Geometry check sheet. Reference: drawing and pictorial views, mm from the part's lowest x, y, z. Round coordinates to 2 decimals unless told otherwise and drop trailing zeros. Order: outer loops, then holes, each group sorted by start corner. A loop starts at its lowest first (then second) coordinate and runs counter-clockwise, first axis right, second up. Notation, with made-up numbers: M -27,68 L 13,68 A18 cw 13,92 Z; hole C -16.75,23.25 d10. An arc over 180 degrees is marked long. Answer as a JSON object with one key per item and string values. Group by question number.
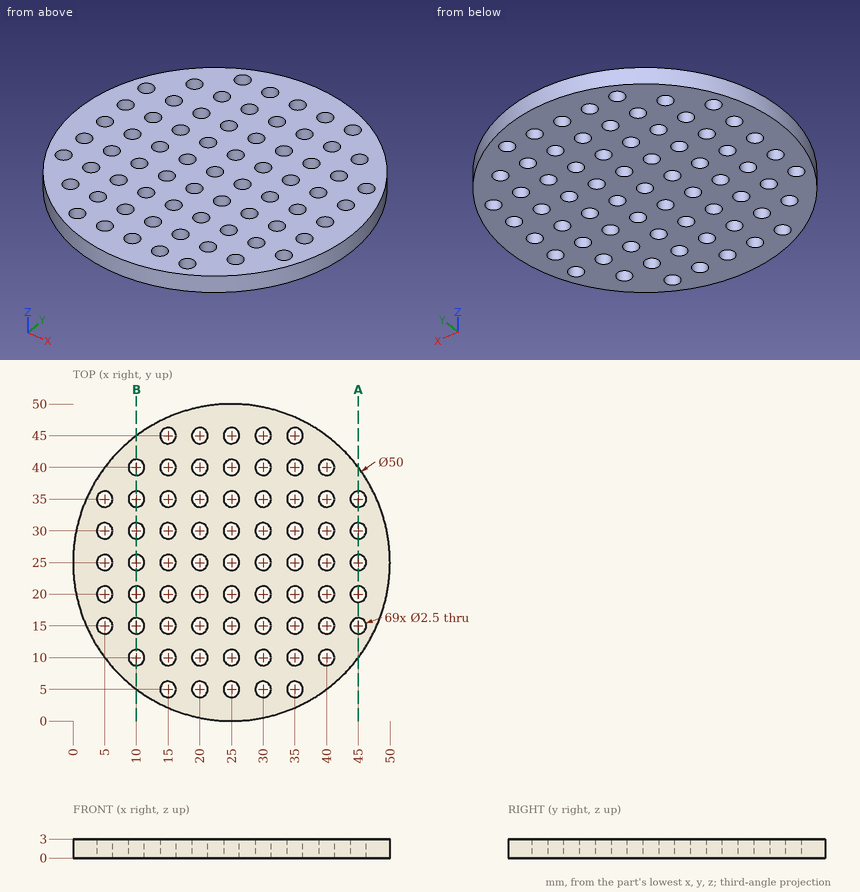
Q1. Cross-section at A-A, the plane x = 45. Record the cut outline in (y, z), then the cut area to 3 significant figures.
Q2. Gauge pin test, flat end, axial feed: pin 1 Ø2 at (x, y) = (35, 45) entering from -Z. Record the tip position at first contact, or that the pin passes through.
Q3. Cross-section at B-B, the plane x = 10. Give the number of separate pieces and of enclosed holes in the cut face, then the cut area to 3 significant figures.
Q4. Thickness scan on line 1 (X direction, y = 45, z = 1.65); line 2 (Y direction, x = 4.5, z = 1.25); line 3 (X direction, y = 44.5, z = 0.7). Record the ranges inside material, lowest first. Write a range as from..to.
Conclusion:
{
 "1": {"outline": "M 10,0 L 13.75,0 L 13.75,3 L 10,3 Z; M 16.25,0 L 18.75,0 L 18.75,3 L 16.25,3 Z; M 21.25,0 L 23.75,0 L 23.75,3 L 21.25,3 Z; M 26.25,0 L 28.75,0 L 28.75,3 L 26.25,3 Z; M 31.25,0 L 33.75,0 L 33.75,3 L 31.25,3 Z; M 36.25,0 L 40,0 L 40,3 L 36.25,3 Z", "area": "52.5 mm2"},
 "2": {"pin 1": "through"},
 "3": {"separate pieces": "8", "enclosed holes": "0", "area": "67.5 mm2"},
 "4": {"line 1": "10..13.75, 16.25..18.75, 21.25..23.75, 26.25..28.75, 31.25..33.75, 36.25..40", "line 2": "10.69..13.85, 16.15..18.85, 21.15..23.85, 26.15..28.85, 31.15..33.85, 36.15..39.31", "line 3": "9.36..13.85, 16.15..18.85, 21.15..23.85, 26.15..28.85, 31.15..33.85, 36.15..40.64"}
}
